from build123d import *

# Parameters (mm, degrees)
SKETCH_1_W          = 10.5
SKETCH_1_H          = 9
EXTRUDE_1_DEPTH     = 0.3
SKETCH_2_R          = 0.125
CUT_EXTRUDE_1_DEPTH = 1.3


with BuildPart() as part:
    # Эскиз1 → Бобышка-Вытянуть1 (new body)
    with BuildSketch(Plane(origin=(0, 0, 0), x_dir=(1, 0, 0), z_dir=(0, 1, 0))):
        Rectangle(SKETCH_1_W, SKETCH_1_H)
    extrude(amount=EXTRUDE_1_DEPTH)

    # Эскиз2 → Вырез-Вытянуть1 (cut, through all)
    with BuildSketch(Plane(origin=(0, 0.3, 0), x_dir=(1, 0, 0), z_dir=(0, 1, 0))):
        with Locations((-3.75, 0.25)):
            Circle(SKETCH_2_R)
        with Locations((-1.25, 0.25)):
            Circle(SKETCH_2_R)
        with Locations((1.25, 0.25)):
            Circle(SKETCH_2_R)
        with Locations((3.75, 0.25)):
            Circle(SKETCH_2_R)
        with Locations((-1.25, -0.25)):
            Circle(SKETCH_2_R)
        with Locations((1.25, -0.25)):
            Circle(SKETCH_2_R)
        with Locations((3.75, -0.25)):
            Circle(SKETCH_2_R)
        with Locations((-3.75, -0.25)):
            Circle(SKETCH_2_R)
    extrude(amount=-CUT_EXTRUDE_1_DEPTH, mode=Mode.SUBTRACT)


solid = part.part
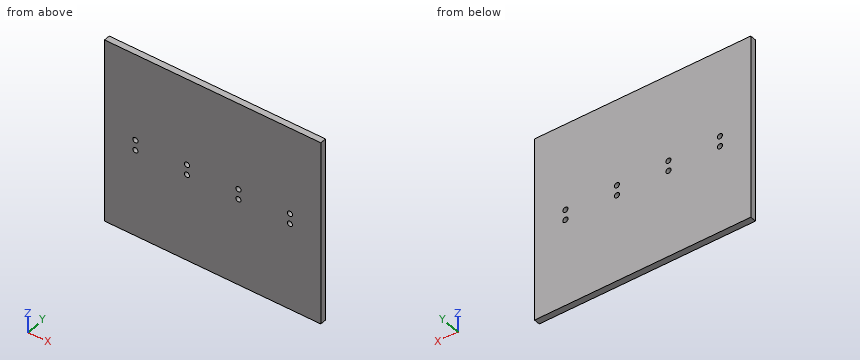
Could you check a few things on this model? Use its own coordinates, in mm. Coordinates: 2 decimals unless noted, no trailing zeros. Order: outer loops, then holes, each group sorted by start corner. A loop starts at its lowest first (then second) coordinate and runs counter-clockwise, first axis right, second up. Notation, with made-up numbers: (-23.75, -31) -> (-4.75, -31) arc R31 cw to (-4.75, 8) -> close; hole circle Ø2 at (72, -23.5). An arc over 180 degrees is marked (long way). One line per question, with ' | ' between items.
Q1. Imagine slicing it at A-A on x = -3.75. Please give me the cut outline in (y, z) (3 decimals), and give its area (3 significant figures).
Return value:
outline: (0, -4.5) -> (0.3, -4.5) -> (0.3, -0.375) -> (0, -0.375) -> close; (0, -0.125) -> (0.3, -0.125) -> (0.3, 0.125) -> (0, 0.125) -> close; (0, 0.375) -> (0.3, 0.375) -> (0.3, 4.5) -> (0, 4.5) -> close | area: 2.55 mm²
Q2. Imagine slicing it at B-B on z = 0.25. Please give me the cut outline in (x, y) (3 decimals).
Return value:
outline: (-5.25, 0) -> (-3.875, 0) -> (-3.875, 0.3) -> (-5.25, 0.3) -> close; (-3.625, 0) -> (-1.375, 0) -> (-1.375, 0.3) -> (-3.625, 0.3) -> close; (-1.125, 0) -> (1.125, 0) -> (1.125, 0.3) -> (-1.125, 0.3) -> close; (1.375, 0) -> (3.625, 0) -> (3.625, 0.3) -> (1.375, 0.3) -> close; (3.875, 0) -> (5.25, 0) -> (5.25, 0.3) -> (3.875, 0.3) -> close
Q3. If I drill on L1, parallel to X at y = 0.1, z = -0.25 (3 decimals); L2, parallel to Z at x = -1.25, y = 0.15 (3 decimals), over which ranges is the centre line in solid material (lowest first)?
Return value:
L1: -5.25 to -3.875, -3.625 to -1.375, -1.125 to 1.125, 1.375 to 3.625, 3.875 to 5.25 | L2: -4.5 to -0.375, -0.125 to 0.125, 0.375 to 4.5
